Read the model definition and answer for the solid it produces. Units are mm, in the model's axes. Face numbers are marked on the shaded views. A direction names the side the tool comes from. Coordinates: 2 decimals unless noted, no trailing zeros. Loops run counter-clockwise (first coordinate to the right, second up) from the corner with the lowest first, then second, coordinate; pieces in that order, holes last. Notation, with made-up numbers: (48.25, 69) -> (93.25, 69) arc R16 ccw to (93.25, 76) -> close; hole circle Ø6 at (21, -3). An arc over 180 degrees is marked (long way). Answer as a JSON object with one key per item and string values. Group by question number.
Q1. This flat-tipped pin is pushed along its axis until it touches: P1, Ø2, axis at x = 1, z = -1, coming from the -Y side. Where does it stop, or does it pass through?
Q2. Determine the mould class of the marked faces 1, 2, 3 and 4 for opening direction Z: released by +Z, released by -Z, zero draft, split by the parting line, or undercut.
Q3. The part is cut by section A-A on x = -1.5. Write down the section's boundary in (y, z), and give its area (3 significant figures).
Q4. For the marked faces 5 and 6, determine the directions among +Z, -Z, +X, -X, +Y, -Y from which every point of the face is accessible in a straight line to the end or side of a thin tool.
Q5. The part is cut by section C-C on z = 0.5. Write down the section's boundary in (x, y), and give its area (3 significant figures).
Q6. The part is cut by section D-D on z = -0.75. Write down the section's boundary in (x, y).
Q7. The part is cut by section B-B on y = 0.85. Write down the section's boundary in (x, z).
Q8. Straight lines are drawn through the part: line 1 along Z through (x, y) = (0.5, 0.6); line 2 along X through (y, z) = (0.75, -2.25); line 3 along X through (y, z) = (0.5, 0.5). For each, find the intervals that lie inside material, in ascending order. Write a range as [from, to].
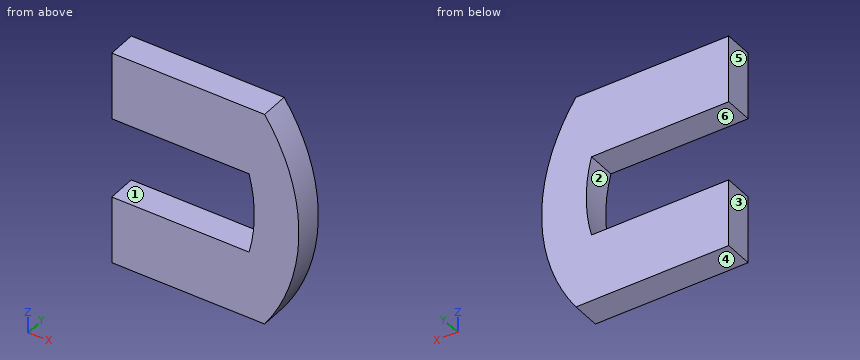
Autodesk Inventor part; units mm, degrees
ref_plane "YZ Plane" through (0, 0, 0) normal (1, 0, 0) x (0, 1, 0)
ref_plane "XZ Plane" through (0, 0, 0) normal (0, 1, 0) x (-1, 0, 0)
ref_plane "XY Plane" through (0, 0, 0) normal (0, 0, 1) x (1, 0, 0)
sketch "Эскиз1" plane through (0, 0, 0) normal (0, 1, 0) x (-1, 0, 0)
  line L0 (2.6545, 3.75) -> (-2.6545, 3.75)
  line L1 (-2.6545, 3.75) -> (-2.6545, -3.75) construction
  line L2 (-2.6545, -3.75) -> (2.6545, -3.75)
  line L3 (2.6545, -3.75) -> (2.6545, 3.75)
  line L4 (3.9547, 0) -> (-5.1453, 0)
  line L5 (0, -5.25) -> (0, 5.25)
  arc A0 (-2.6545, 3.75) -> (-2.6545, -3.75) centre (2.6547, 0) ccw
  point P0 (0, 0)
  dimension "d0" = 5.309
  dimension "d1" = 7.5
  dimension "d2" = 6.5
extrude "Выдавливание1" add sketch "Эскиз1" along normal blind 1
sketch "Эскиз2" plane through (0, 1, 0) normal (0, 1, 0) x (1, 0, 0)
  line L0 (-2.6545, 3.75) -> (-2.6545, -3.75)
  line L1 (-2.6545, -1.4) -> (2.1155, -1.4)
  line L2 (2.1155, -1.4) -> (2.1155, 1.4) construction
  line L3 (2.1155, 1.4) -> (-2.6545, 1.4)
  line L4 (-2.6545, 1.4) -> (-2.6545, -1.4)
  line L5 (-4.6131, 0) -> (5.255, 0)
  arc A0 (2.1155, -1.4) -> (2.1155, 1.4) centre (-3.2033, 0) ccw
  point P0 (0, 0)
  dimension "d5" = 4.77
  dimension "d6" = 2.8
  dimension "d7" = 5.5
extrude "Выдавливание2" cut sketch "Эскиз2" against normal through all
properties part number "BUTTON_TOP"
Final values:
{
 "1": {"P1": "stops at y = 0"},
 "2": {"face 1": "undercut", "face 2": "undercut", "face 3": "zero draft", "face 4": "released by -Z"},
 "3": {"outline": "(0, -3.75) -> (1, -3.75) -> (1, -1.4) -> (0, -1.4) -> close; (0, 1.4) -> (1, 1.4) -> (1, 3.75) -> (0, 3.75) -> close", "area": "4.70 mm2"},
 "4": {"face 5": "+Z, -Z, -X, +Y, -Y", "face 6": "-X, +Y, -Y"},
 "5": {"outline": "(2.27, 0) -> (3.83, 0) -> (3.83, 1) -> (2.27, 1) -> close", "area": "1.55 mm2"},
 "6": {"outline": "(2.25, 0) -> (3.8, 0) -> (3.8, 1) -> (2.25, 1) -> close"},
 "7": {"outline": "(-2.65, -3.75) -> (2.65, -3.75) arc R6.5 ccw to (2.65, 3.75) -> (-2.65, 3.75) -> (-2.65, 1.4) -> (2.12, 1.4) arc R5.5 cw to (2.12, -1.4) -> (-2.65, -1.4) -> close"},
 "8": {"line 1": "z = [-3.75, -1.4], [1.4, 3.75]", "line 2": "x = [-2.65, 3.44]", "line 3": "x = [2.27, 3.83]"}
}
